Autodesk Inventor part; units mm, degrees
ref_plane "YZ Plane" through (0, 0, 0) normal (1, 0, 0) x (0, 1, 0)
ref_plane "XZ Plane" through (0, 0, 0) normal (0, 1, 0) x (-1, 0, 0)
ref_plane "XY Plane" through (0, 0, 0) normal (0, 0, 1) x (1, 0, 0)
sketch "Sketch1" plane through (0, 0, 0) normal (0, 1, 0) x (-1, 0, 0)
  line L0 (0, 0) -> (25, 0)
  line L1 (25, 0) -> (25, -42)
  line L2 (25, -42) -> (0, -42)
  line L3 (0, -42) -> (0, 0)
  line L4 (22, 0) -> (3, 0)
  line L5 (3, 0) -> (3, 8)
  line L6 (3, 8) -> (22, 8)
  line L7 (22, 8) -> (22, 0)
  point P0 (22, 4)
  dimension "d0" = 19
  dimension "d1" = 3
  dimension "d2" = 3
  dimension "d3" = 42
  dimension "d4" = 25
  dimension "d27" = 8
extrude "Extrusion1" add sketch "Sketch1" along normal blind 5
sketch "Sketch2" plane through (0, 5, 0) normal (0, 1, 0) x (1, 0, 0)
  line L0 (-20, 5) -> (-5, 5)
  line L1 (-5, 5) -> (-5, 15)
  line L2 (-5, 15) -> (-20, 15)
  line L3 (-20, 15) -> (-20, 5)
  line L4 (-25, 0) -> (-22, 0)
  line L5 (-25, 42) -> (-25, 0)
  line L6 (0, 0) -> (0, 42)
  dimension "d7" = 5
  dimension "d8" = 10
  dimension "d25" = 5
  dimension "d26" = 5
extrude "Extrusion2" add sketch "Sketch2" along normal blind 7
sketch "Sketch3" plane through (0, 0, 0) normal (0, -1, 0) x (1, 0, 0)
  circle A0 centre (-1.5, -7.5) radius 1
  line L0 (-3, 0) -> (0, 0)
  line L1 (0, 0) -> (0, -42)
  circle A1 centre (-23.5, -8.5) radius 1
  line L2 (-25, 0) -> (-22, 0)
  line L3 (-25, -42) -> (-25, 0)
  dimension "d13" = 2
  dimension "d14" = 7.5
  dimension "d15" = 1.5
  dimension "d16" = 2
  dimension "d17" = 8.5
  dimension "d18" = 1.5
extrude "Extrusion3" cut sketch "Sketch3" against normal blind 7
thread "Thread1"
thread "Thread2"
sketch "Sketch4" plane through (0, 0, 0) normal (0, -1, 0) x (1, 0, 0)
  line L0 (-3.66, 7.1394) -> (-3.66, 2.0183)
  line L1 (-3.66, 2.0183) -> (-7.1475, 2.0183)
  line L2 (-7.1475, 5.8905) -> (-7.1475, 7.1394)
  line L3 (-7.1475, 7.1394) -> (-3.66, 7.1394)
  line L4 (-7.1475, 5.8905) -> (-8.5429, 2.0183)
  line L5 (-8.5429, 2.0183) -> (-10.2962, 2.0183)
  line L6 (-10.2962, 2.0183) -> (-12.2596, 4.8754)
  line L7 (-12.2596, 4.8754) -> (-12.2596, 7.1394)
  line L8 (-12.2596, 7.1394) -> (-10.6175, 7.1394)
  line L9 (-10.6175, 7.1394) -> (-10.6175, 4.8754)
  line L10 (-10.6175, 4.8754) -> (-8.9607, 4.8754)
  line L11 (-8.9607, 4.8754) -> (-8.9607, 7.1394)
  line L12 (-8.9607, 7.1394) -> (-7.1475, 7.1394)
  line L13 (-12.2596, 4.8754) -> (-12.2596, 2.0183)
  line L14 (-14.9412, 1.77) -> (-14.9412, 3.503)
  line L15 (-13.1457, 3.503) -> (-13.1457, 6.1648)
  line L16 (-13.1457, 6.1648) -> (-14.9412, 6.1648)
  line L17 (-14.9412, 6.1648) -> (-14.9412, 7.1394)
  line L18 (-12.2596, 7.1394) -> (-14.9412, 7.1394)
  line L19 (-12.2596, 2.0183) -> (-12.2596, 1.8295)
  line L20 (-14.9412, 3.503) -> (-14.9412, 6.1648)
  line L21 (-7.1475, 2.0183) -> (-7.1475, 4.4084)
  line L22 (-7.1475, 4.4084) -> (-4.6775, 4.4084)
  line L23 (-4.6775, 4.4084) -> (-4.6775, 5.2007)
  line L24 (-4.6775, 5.2007) -> (-7.1475, 5.2007)
  line L25 (-7.1475, 5.2007) -> (-7.1475, 5.8905)
  line L26 (-4.6775, 3.503) -> (-4.6775, 2.6365)
  line L27 (-4.6775, 2.6365) -> (-6.5324, 2.6365)
  line L28 (-6.5324, 2.6365) -> (-6.5324, 3.503)
  line L29 (-6.5324, 3.503) -> (-4.6775, 3.503)
  line L30 (-4.66, 5.8905) -> (-6.5324, 5.8905)
  line L31 (-6.5324, 5.8905) -> (-6.5324, 6.7449)
  line L32 (-6.5324, 6.7449) -> (-4.9174, 6.7449)
  line L33 (-4.9174, 6.7449) -> (-4.66, 5.8905)
  line L34 (-14.9412, 1.77) -> (-16.3182, 1.77)
  line L35 (-16.3182, 1.77) -> (-16.3182, 7.1394)
  line L36 (-16.3182, 7.1394) -> (-14.9412, 7.1394)
  line L37 (-18.5068, 5.8905) -> (-16.4834, 4.2767)
  line L38 (-16.4834, 4.2767) -> (-19.3704, 1.77)
  line L39 (-19.3704, 1.77) -> (-17.9269, 1.77)
  line L40 (-17.9269, 1.77) -> (-16.3182, 3.1668)
  line L41 (-18.5068, 5.8905) -> (-20.0727, 7.1394)
  line L42 (-20.0727, 7.1394) -> (-18.5068, 7.1394)
  line L43 (-16.3182, 5.8905) -> (-18.5068, 7.1394)
  line L44 (-9.0583, 2.869) -> (-10.6175, 2.869)
  line L45 (-10.6175, 2.869) -> (-10.6175, 3.7284)
  line L46 (-10.6175, 3.7284) -> (-9.0583, 3.7284)
  line L47 (-9.0583, 3.7284) -> (-9.0583, 2.869)
  line L48 (-14.0417, 3.5591) -> (-14.15, 1.8295)
  line L49 (-12.2596, 1.8295) -> (-14.15, 1.8295)
  line L50 (-14.0452, 3.503) -> (-13.1457, 3.503)
  line L51 (-2.7778, -34.9531) -> (-2.7778, -41.136)
  line L52 (-2.7778, -41.136) -> (-8.4213, -41.136)
  line L53 (-8.4213, -41.136) -> (-8.4213, -39.4983)
  line L54 (-8.4213, -39.4983) -> (-4.4166, -39.4983)
  line L55 (-4.4166, -39.4983) -> (-4.4166, -38.0343)
  line L56 (-4.4166, -38.0343) -> (-9.0583, -38.0343)
  line L57 (-9.0583, -38.0343) -> (-8.4213, -36.2667)
  line L58 (-8.4213, -36.2667) -> (-4.4166, -36.2667)
  line L59 (-4.4166, -36.2667) -> (-4.4166, -33.2701)
  line L60 (-4.4166, -33.2701) -> (-2.3323, -33.7168)
  line L61 (-2.3323, -33.7168) -> (-2.7778, -34.9531)
  line L62 (-10.176, -41.136) -> (-9.8379, -32.7739)
  line L63 (-9.8379, -32.7739) -> (-12.2596, -33.2701)
  line L64 (-12.2596, -33.2701) -> (-11.8606, -36.5207)
  line L65 (-11.8606, -36.5207) -> (-13.5954, -36.9549)
  line L66 (-13.5954, -36.9549) -> (-14.8005, -36.5207)
  line L67 (-14.8005, -36.5207) -> (-15.3476, -34.335)
  line L68 (-15.3476, -34.335) -> (-15.6141, -33.2701)
  line L69 (-15.6141, -33.2701) -> (-16.8071, -32.8402)
  line L70 (-16.8071, -32.8402) -> (-16.8627, -34.2134)
  line L71 (-16.8627, -34.2134) -> (-16.9559, -36.5207)
  line L72 (-16.9559, -36.5207) -> (-16.6555, -37.7209)
  arc A0 (-15.6141, -37.7209) -> (-16.6555, -37.7209) centre (-16.1348, -39.8012) ccw
  line L73 (-15.6141, -37.7209) -> (-14.4216, -38.0343)
  line L74 (-14.4216, -38.0343) -> (-16.3182, -39.1953)
  line L75 (-16.3182, -39.1953) -> (-16.9559, -41.136)
  line L76 (-16.9559, -41.136) -> (-10.176, -41.136)
  circle A1 centre (-13.2048, -39.1953) radius 1.2392
  circle A2 centre (-18.8951, -37.3841) radius 1.5485
  line L77 (-21.1041, -32.8402) -> (-20.4436, -35.3671)
  line L78 (-20.4436, -35.3671) -> (-22.4923, -35.3671)
  line L79 (-22.4923, -35.3671) -> (-22.4923, -32.8402)
  line L80 (-22.4923, -32.8402) -> (-22.059, -32.8402)
  line L81 (-22.059, -32.8402) -> (-22.059, -34.4396)
  line L82 (-22.059, -34.4396) -> (-21.468, -34.4396)
  line L83 (-21.468, -34.4396) -> (-21.1041, -32.8402)
  line L84 (-23.4723, -32.8402) -> (-24.287, -32.8402)
  line L85 (-24.287, -32.8402) -> (-24.287, -39.8012)
  line L86 (-24.287, -39.8012) -> (-24.9664, -39.8012)
  line L87 (-24.9664, -39.8012) -> (-24.538, -41.4401)
  line L88 (-24.538, -41.4401) -> (-17.5177, -41.4401)
  line L89 (-17.5177, -41.4401) -> (-17.9667, -39.7224)
  line L90 (-17.9667, -39.7224) -> (-23.8797, -39.7224)
  line L91 (-23.8797, -39.7224) -> (-23.4723, -32.8402)
  point P0 (0, 0)
extrude "Extrusion4" add sketch "Sketch4" along normal blind 1
properties part number "Head"
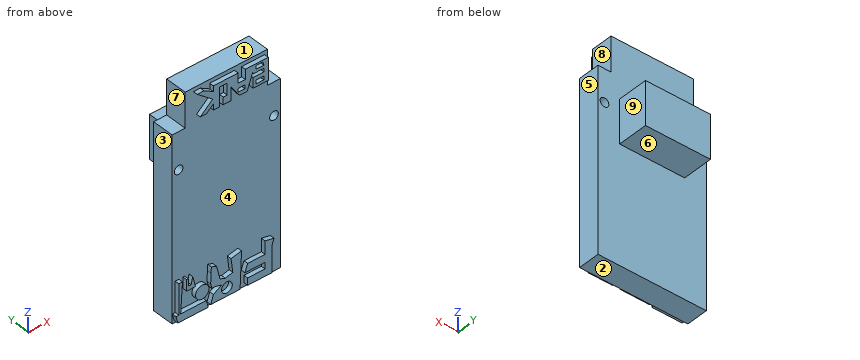
Verification items for the finished model (mm, model axes). Face numbers are marked on the shaded views. A direction names the side the tool comes from. Coordinates: 2 decimals unless noted, no trailing zeros. Write each loop counter-clockwise with the first axis right and the second up, starting at its lowest first coordinate (ties: lowest second). Pieces come first, ordered by that corner, then holes. Notation, with made-up numbers: M 83,-40 L 113,-40 A26 cw 113,-23 Z; hole C 75,-39 d7. An arc over 180 degrees is marked long. One line per item, written item: value.
Item 1: Scan lines: line 1 along Z through (x, y) = (-23.5, 3.55); line 2 along Z through (x, y) = (-17.5, 7.5); line 3 along Y through (x, z) = (-3.75, 4). Record each from-to range of solid material in increasing order.
Check sheet entries:
line 1: z = -42 to -9.5, -7.5 to 0
line 2: z = -15 to -5
line 3: y = -1 to 5
Item 2: Section check D-D, the plane y = 10.5. Record the boundary of the cut face in (x, z), plus the area to 3 significant figures.
Check sheet entries:
outline: M -20,-15 L -5,-15 L -5,-5 L -20,-5 Z
area: 150 mm^2
Item 3: Section check B-B, the plane y = 2.75. Record the boundary of the cut face in (x, z), plus the area to 3 significant figures.
Check sheet entries:
outline: M -25,-42 L 0,-42 L 0,0 L -3,0 L -3,8 L -22,8 L -22,0 L -25,0 Z; hole C -23.5,-8.5 d2; hole C -1.5,-7.5 d2
area: 1,200 mm^2
Item 4: Access from +Z, -Z, +X, -X, +Y, -Y to the whole of each face (thin tool, end or side, straight path). Record for the marked faces 5, 6, 7, 8 and 9.
Check sheet entries:
face 5: +Z, -Z, +X, +Y, -Y
face 6: -Z, +X, -X, +Y
face 7: +Z, -X, +Y, -Y
face 8: +Z, +X, +Y, -Y
face 9: +Z, -Z, +X, +Y
Item 5: Section check C-C, the plane z = -6. Record the boundary of the cut face in (x, y), plus the area to 3 significant figures.
Check sheet entries:
outline: M -25,0 L 0,0 L 0,5 L -5,5 L -5,12 L -20,12 L -20,5 L -25,5 Z
area: 230 mm^2
Item 6: Gauge pin test, flat ends, axial feed: pin 1 Ø5 at (x, z) = (-3.5, -35) entering from +Y; pin 2 Ø6 at (y, z) = (10.5, -31) entering from +X; pin 3 Ø0.8 at (x, y) = (-13, -0.5) entering from +Z; pin 4 Ø0.5 at (x, y) = (-4, -0.5) entering from -Z. Record the tip position at first contact, or that the pin passes through.
Check sheet entries:
pin 1: stops at y = 5
pin 2: passes through
pin 3: stops at z = 7.14
pin 4: stops at z = -41.14
Item 7: Section check A-A, the plane x = -1.5. Record the boundary of the cut face in (y, z).
Check sheet entries:
outline: M 0,-42 L 5,-42 L 5,-8.5 L 0,-8.5 Z; M 0,-6.5 L 5,-6.5 L 5,0 L 0,0 Z
Item 8: Mould release check, pull along Z, two halves, no side actions. Record for the marked faces 1, 2, 3 and 4: pulls with the +Z half, pulls with the -Z half, needs draft (parallel to the pull), parting line crosses it, or undercut.
Check sheet entries:
face 1: pulls with the +Z half
face 2: pulls with the -Z half
face 3: needs draft
face 4: undercut
